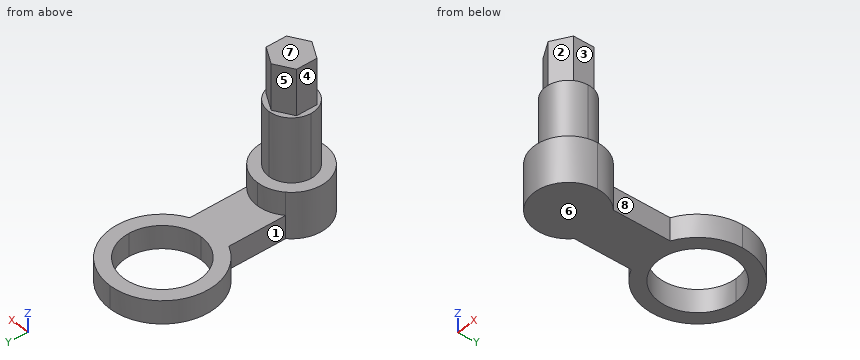
from build123d import *

# Parameters (mm, degrees)
F1_DEPTH = 5
F2_DEPTH = 10
F3_DEPTH = 24
F4_DEPTH = 34


with BuildPart() as f1:
    # F0 (on Top) → F1 (new body)
    with BuildSketch(Plane.XY):
        with BuildLine():
            ThreePointArc((0, 40), (-11.2103927734, 31.0645845405), (-5, 18.1438424114))
            Line((-5, 18.1438424114), (-5, 19.8613982648))
            Line((-5, 19.8613982648), (0, 19.8613982648))
            Line((0, 19.8613982648), (0, 20))
            ThreePointArc((0, 20), (-8.5, 28.5), (0, 37))
            Line((0, 37), (0, 40))
        make_face()
        with BuildLine():
            Line((5, 19.8613982648), (5, 18.1438424114))
            ThreePointArc((5, 18.1438424114), (9.7403798694, 22.3864903697), (11.5, 28.5))
            ThreePointArc((11.5, 28.5), (8.1317279836, 36.6317279836), (0, 40))
            Line((0, 40), (0, 37))
            ThreePointArc((0, 37), (6.0104076401, 34.5104076401), (8.5, 28.5))
            ThreePointArc((8.5, 28.5), (6.0104076401, 22.4895923599), (0, 20))
            Line((0, 20), (0, 19.8613982648))
            Line((0, 19.8613982648), (5, 19.8613982648))
        make_face()
        with BuildLine():
            ThreePointArc((0, 17), (2.5645845405, 17.2896072266), (5, 18.1438424114))
            Line((5, 18.1438424114), (5, 19.8613982648))
            Line((5, 19.8613982648), (0, 19.8613982648))
            Line((0, 19.8613982648), (0, 17))
        make_face()
        with BuildLine():
            Line((-5, 19.8613982648), (-5, 18.1438424114))
            ThreePointArc((-5, 18.1438424114), (-2.5645845405, 17.2896072266), (0, 17))
            Line((0, 17), (0, 19.8613982648))
            Line((0, 19.8613982648), (-5, 19.8613982648))
        make_face()
        with BuildLine():
            Line((-5, 18.1438424114), (-5, 5.5901699437))
            ThreePointArc((-5, 5.5901699437), (-2.6761656733, 7.0062926922), (0, 7.5))
            Line((0, 7.5), (0, 17))
            ThreePointArc((0, 17), (-2.5645845405, 17.2896072266), (-5, 18.1438424114))
        make_face()
        with BuildLine():
            ThreePointArc((0, 7.5), (2.6761656733, 7.0062926922), (5, 5.5901699437))
            Line((5, 5.5901699437), (5, 18.1438424114))
            ThreePointArc((5, 18.1438424114), (2.5645845405, 17.2896072266), (0, 17))
            Line((0, 17), (0, 7.5))
        make_face()
    extrude(amount=F1_DEPTH)

    # F0 (on Top) → F2 (join)
    with BuildSketch(Plane.XY):
        with BuildLine():
            Line((5, 0), (5, 5.5901699437))
            ThreePointArc((5, 5.5901699437), (2.6761656733, 7.0062926922), (0, 7.5))
            Line((0, 7.5), (0, 5))
            ThreePointArc((0, 5), (3.5355339059, 3.5355339059), (5, 0))
        make_face()
        with BuildLine():
            ThreePointArc((-5, 5.5901699437), (-3.0618621785, -6.8465319688), (7.5, 0))
            ThreePointArc((7.5, 0), (6.8465319688, 3.0618621785), (5, 5.5901699437))
            Line((5, 5.5901699437), (5, 0))
            ThreePointArc((5, 0), (0, -5), (-5, 0))
            Line((-5, 0), (-5, 5.5901699437))
        make_face()
        with BuildLine():
            ThreePointArc((0, 7.5), (-2.6761656733, 7.0062926922), (-5, 5.5901699437))
            Line((-5, 5.5901699437), (-5, 0))
            ThreePointArc((-5, 0), (-3.5355339059, 3.5355339059), (0, 5))
            Line((0, 5), (0, 7.5))
        make_face()
    extrude(amount=F2_DEPTH)

    # F0 (on Top) → F3 (join)
    with BuildSketch(Plane.XY):
        with BuildLine():
            Line((3.897114317, 0), (5, 0))
            ThreePointArc((5, 0), (3.5355339059, 3.5355339059), (0, 5))
            Line((0, 5), (0, 4.5))
            Line((0, 4.5), (3.897114317, 2.25))
            Line((3.897114317, 2.25), (3.897114317, 0))
        make_face()
        with BuildLine():
            ThreePointArc((-5, 0), (0, -5), (5, 0))
            Line((5, 0), (3.897114317, 0))
            Line((3.897114317, 0), (3.897114317, -2.25))
            Line((3.897114317, -2.25), (0, -4.5))
            Line((0, -4.5), (-3.897114317, -2.25))
            Line((-3.897114317, -2.25), (-3.897114317, 0))
            Line((-3.897114317, 0), (-5, 0))
        make_face()
        with BuildLine():
            ThreePointArc((0, 5), (-3.5355339059, 3.5355339059), (-5, 0))
            Line((-5, 0), (-3.897114317, 0))
            Line((-3.897114317, 0), (-3.897114317, 2.25))
            Line((-3.897114317, 2.25), (0, 4.5))
            Line((0, 4.5), (0, 5))
        make_face()
    extrude(amount=F3_DEPTH)

    # F0 (on Top) → F4 (join)
    with BuildSketch(Plane.XY):
        Polygon((3.897114317, 2.25), (0, 4.5), (0, 0), align=None)
        Polygon((0, 0), (3.897114317, 0), (3.897114317, 2.25), align=None)
        Polygon((3.897114317, -2.25), (3.897114317, 0), (0, 0), align=None)
        Polygon((3.897114317, -2.25), (0, 0), (0, -4.5), align=None)
        Polygon((0, -4.5), (0, 0), (-3.897114317, -2.25), align=None)
        Polygon((0, 0), (-3.897114317, 0), (-3.897114317, -2.25), align=None)
        Polygon((-3.897114317, 2.25), (-3.897114317, 0), (0, 0), align=None)
        Polygon((0, 0), (0, 4.5), (-3.897114317, 2.25), align=None)
    extrude(amount=F4_DEPTH)


solid = f1.part
Part model, mm, in its own coordinate system. Face numbers are marked on the shaded views. A direction names the side the tool comes from. Give positions to 0.01 mm unless a question says otherwise; leave off trailing zeros. Write each loop counter-clockwise with the first axis right and the second up, starting at its lowest first coordinate (ties: lowest second). Pieces come first, ordered by that corner, then holes.
1) Which spindle directions (+Z, -Z, +X, -X, +Y, -Y) get a long thin tool onto all of the face, cutting with end or side? Do the marked faces 4, 5, 6, 7 and 8. Say none if no direction does.
Resolved:
face 4: +Z, -X, +Y, -Y
face 5: +Z, -X, +Y
face 6: -Z, +X, -X, +Y, -Y
face 7: +Z, +X, -X, +Y, -Y
face 8: +Z, -Z, +X
2) Cut at D-D on x = 2.75. Write the cut outline in (y, z), then the cut area to 3 significant figures.
Resolved:
outline: (-6.98, 0) - (20.46, 0) - (20.46, 5) - (6.98, 5) - (6.98, 10) - (4.18, 10) - (4.18, 24) - (2.91, 24) - (2.91, 34) - (-2.91, 34) - (-2.91, 24) - (-4.18, 24) - (-4.18, 10) - (-6.98, 10) - close; (36.54, 0) - (39.67, 0) - (39.67, 5) - (36.54, 5) - close
area: 398 mm2
3) Two-plate mould, pull along Y, no slides. Class the marked faces 1, 2 and 3: released by +Y, released by -Y, zero draft, split by the parting line, or undercut.
Resolved:
face 1: undercut
face 2: released by -Y
face 3: zero draft
4) Cut at B-B on y = 35. Write the cut outline in (x, z).
Resolved:
outline: (-9.49, 0) - (-5.48, 0) - (-5.48, 5) - (-9.49, 5) - close; (5.48, 0) - (9.49, 0) - (9.49, 5) - (5.48, 5) - close
5) Cut at C-C on z = 3. Write the cut outline in (x, y).
Resolved:
outline: (-5, 5.59) arc R7.5 ccw (long way) to (5, 5.59) - (5, 18.14) arc R11.5 ccw (long way) to (-5, 18.14) - close; hole circle Ø17 at (0, 28.5)
6) Probe L1, parallel to Z at x = -4.5, y = 9; L2, parallel to Z at x = 2.25, y = -4; L3, parallel to X at y = 33, z = 2.5. List the from-to ranges inside material, lowest first.
Resolved:
L1: z = 0 to 5
L2: z = 0 to 24
L3: x = -10.58 to -7.21, 7.21 to 10.58
7) Cut at A-A on x = 6.25. Write the cut outline in (y, z).
Resolved:
outline: (-4.15, 0) - (4.15, 0) - (4.15, 10) - (-4.15, 10) - close; (18.85, 0) - (22.74, 0) - (22.74, 5) - (18.85, 5) - close; (34.26, 0) - (38.15, 0) - (38.15, 5) - (34.26, 5) - close
8) Pin check, flat tips, straight feed: pin 1 (12 mm diameter, centred on y = 1, z = 15, fed in from +X); pin 2 (3.5 mm diameter, centred on y = 1, z = 29, fed in from +X); pin 3 (7 mm diameter, centred on x = 4.5, y = 18.5, fed in from +Z). Stop position of each tip, or through.
Resolved:
pin 1: stops at x = 7.5
pin 2: stops at x = 3.9
pin 3: stops at z = 5
